Autodesk Inventor part; units mm, degrees
ref_plane "YZ Plane" through (0, 0, 0) normal (1, 0, 0) x (0, 1, 0)
ref_plane "XZ Plane" through (0, 0, 0) normal (0, 1, 0) x (-1, 0, 0)
ref_plane "XY Plane" through (0, 0, 0) normal (0, 0, 1) x (1, 0, 0)
sketch "スケッチ1" plane through (0, 0, 0) normal (0, 0, 1) x (1, 0, 0)
  line L0 (-30, 20) -> (30, 20)
  line L1 (30, 20) -> (30, -20)
  line L2 (30, -20) -> (-30, -20)
  line L3 (-30, -20) -> (-30, 20)
  line L4 (-30, 20) -> (30, -20) construction
  line L5 (30, 20) -> (-30, -20) construction
  point P0 (0, 0)
  dimension "d0" = 60
  dimension "d1" = 40
extrude "押し出し1" add sketch "スケッチ1" along normal blind 4
sketch "スケッチ2" plane through (0, 0, 4) normal (0, 0, 1) x (1, 0, 0)
  line L0 (-10, 55) -> (10, 55)
  line L1 (10, 55) -> (10, -45)
  line L2 (10, -45) -> (-10, -45)
  line L3 (-10, -45) -> (-10, 55)
  point P0 (0, 0)
  dimension "d4" = 20
  dimension "d5" = 100
  dimension "d6" = 10
  dimension "d7" = 55
extrude "押し出し2" add sketch "スケッチ2" against normal blind 4
fillet "フィレット1" radius 10 4 edges at (10, 55, 2) (-10, 55, 2) (10, -45, 2) (-10, -45, 2)
fillet "フィレット2" radius 2 22 edges at (10, 32.5001, 4) (-10, 32.5001, 4) (-7.0711, 52.0711, 4) (7.0711, 52.0711, 4) (20, 20, 4) (30, 0, 4) (20, -20, 4) (-7.0711, -42.0711, 4) (7.0711, -42.0711, 4) (-10, -27.5001, 4) (10, -27.5, 4) (-20, -20, 4) (-30, 0, 4) (-20, 20, 4) (-30, 20, 2) (-10, 20, 2) (-30, -20, 2) (-10, -20, 2) (10, -20, 2) (30, -20, 2) (30, 20, 2) (10, 20, 2)
sketch "スケッチ3" plane through (0, 0, 4) normal (0, 0, 1) x (1, 0, 0)
  arc A0 (10, 45) -> (-10, 45) centre (0, 45) ccw
  arc A1 (-10, -35) -> (10, -35) centre (0, -35) ccw
  point P0 (0, 0)
  dimension "d12" = 0
  dimension "d13" = 0
hole "穴1" at (0, -35, 4) at (0, 45, 4) direction (0, 0, -1) diameter 6 end through all
properties part number "joy_mount_T"
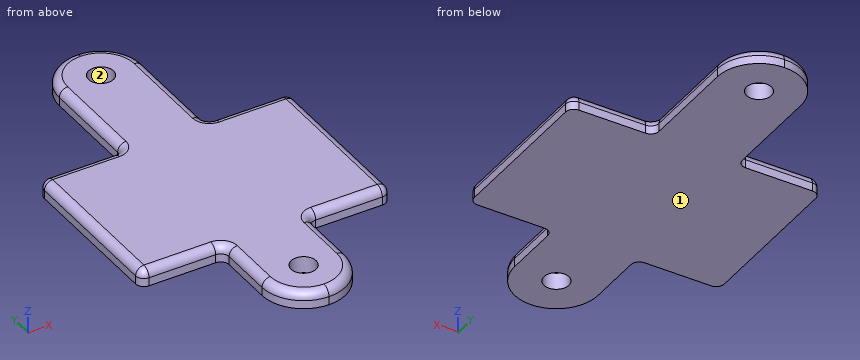
Build history of the part. All positions in model axes, mm. Face numbers are marked on the shaded views. Round coordinates to 2 decimals unless told otherwise and drop trailing zeros. Loops run counter-clockwise (first coordinate to the right, second up) from the corner with the lowest first, then second, coordinate; pieces in that order, holes last.
Item 1: Saw through at B-B (x = -18.5). List the corners of the cut face in (y, z), then the cut area to 3 significant figures.
Item 2: Saw through at C-C (y = 37). List the corners of the cut face in (x, z).
Item 3: Two-plate mould, pull along Y, no slides. Class the marked faces 1 and 2: released by +Y, released by -Y, zero draft, split by the parting line, or undercut.
Item 4: Saw through at A-A (z = 1.1). State how many separate pieces and enclosed holes the cut face has, then the cut area to 3 significant figures.
Item 5: Pin check, flat tips, straight feed: P1, Ø1.6, axis at y = -29, z = 0.5, coming from the -X side; P2, Ø2, axis at x = 2, z = 3.5, coming from the +Y side; P3, Ø0.6, axis at x = -17, z = 1.5, coming from the -Y side. Stop position of each tip, or through.
Item 6: Drill centre lines: line 1 along Y through (x, z) = (0, 1.65); line 2 along Y through (x, z) = (0, 2.9); line 3 along X through (y, z) = (45, 1.35). Where is each one in solid material? Low to high.
Worked answers:
1. outline: (-20, 0) - (20, 0) - (20, 2) arc R2 ccw to (18, 4) - (-18, 4) arc R2 ccw to (-20, 2) - close
1. area: 158 mm2
2. outline: (-10, 0) - (10, 0) - (10, 2) arc R2 ccw to (8, 4) - (-8, 4) arc R2 ccw to (-10, 2) - close
3. face 1: zero draft
3. face 2: undercut
4. separate pieces: 1
4. enclosed holes: 2
4. area: 3,460 mm2
5. P1: stops at x = -10
5. P2: stops at y = 54.78
5. P3: stops at y = -20
6. line 1: y = -45 to -38, -32 to 42, 48 to 55
6. line 2: y = -44.79 to -38, -32 to 42, 48 to 54.79
6. line 3: x = -10 to -3, 3 to 10
